The figure shows three views and two pictorial views of one solid part (mm, origin at its lowest corner). Answer the questions. Round coordinates to 2 decimals unless told otherwise and drop trailing zeros. Write each loop counter-clockwise with the first axis right and the second up, starting at its lowest first coordinate (ties: lowest second). Pieces come first, ordered by that corner, then holes. Notation, with made-up numbers: (29, 78) - (60, 78) arc R21 ccw to (60, 94) - close; hole circle Ø5 at (-29, 44.5). An arc over 180 degrees is marked (long way). Answer as CSV lines item,"result". Start each with the question number.
Item 1: A cutting plane is placed at B-B on y = 75. Determine the outline of the cut face in (x, z), and give its area (3 significant figures).
Item 2: A cutting plane is placed at D-D on x = 50. Determine the outline of the cut face in (y, z), and give its area (3 significant figures).
Item 3: Straight lines are drawn through the part: line 1 along X through (y, z) = (75, 1.55); line 2 along Y through (x, z) = (85, 1.3); line 3 along Y through (x, z) = (15, 2.65). For each, find the intervals that lie inside material, in ascending order. Write a range as [from, to].
Item 4: A cutting plane is placed at A-A on z = 4.25. Determine the outline of the cut face in (x, y), and give its area (3 significant figures).
Item 5: Flat-ended cylindrical pins translate along their axes: pin 1 (5.5 mm diameter, centred on x = 15, y = 5, fed in from +Z); pin 2 (3 mm diameter, centred on x = 85, y = 5, fed in from -Z). Find the tip coordinate at first contact, or state that the pin passes through.
Item 6: A cutting plane is placed at C-C on x = 85. Determine the outline of the cut face in (y, z), and give its area (3 significant figures).
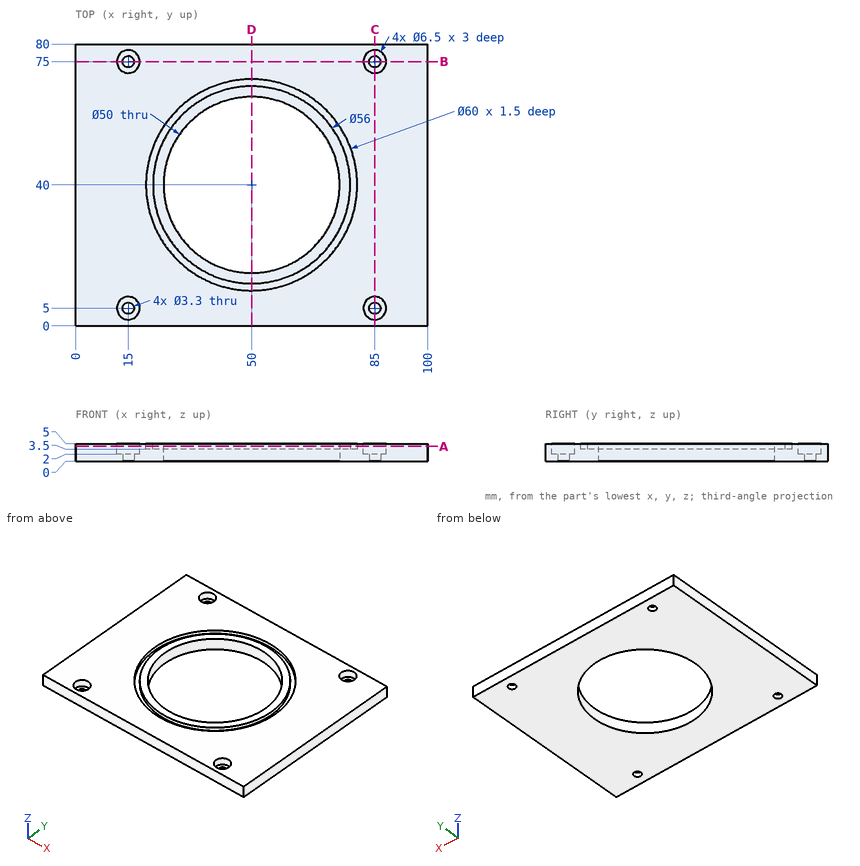
Geometry says:
1,outline,"(0, 0) - (13.35, 0) - (13.35, 2) - (11.75, 2) - (11.75, 5) - (0, 5) - close; (16.65, 0) - (83.35, 0) - (83.35, 2) - (81.75, 2) - (81.75, 5) - (18.25, 5) - (18.25, 2) - (16.65, 2) - close; (86.65, 0) - (100, 0) - (100, 5) - (88.25, 5) - (88.25, 2) - (86.65, 2) - close"
1,area,"448 mm^2"
2,outline,"(0, 0) - (15, 0) - (15, 5) - (12, 5) - (12, 3.5) - (10, 3.5) - (10, 5) - (0, 5) - close; (65, 0) - (80, 0) - (80, 5) - (70, 5) - (70, 3.5) - (68, 3.5) - (68, 5) - (65, 5) - close"
2,area,"144 mm^2"
3,line 1,"x = [0, 13.35], [16.65, 83.35], [86.65, 100]"
3,line 2,"y = [0, 3.35], [6.65, 73.35], [76.65, 80]"
3,line 3,"y = [0, 1.75], [8.25, 71.75], [78.25, 80]"
4,outline,"(0, 0) - (100, 0) - (100, 80) - (0, 80) - close; circle Ø56 at (50, 40); hole circle Ø6.5 at (15, 5); hole circle Ø6.5 at (15, 75); hole circle Ø60 at (50, 40); hole circle Ø50 at (50, 40); hole circle Ø6.5 at (85, 5); hole circle Ø6.5 at (85, 75)"
4,area,"5,540 mm^2"
5,pin 1,"stops at z = 2"
5,pin 2,"passes through"
6,outline,"(0, 0) - (3.35, 0) - (3.35, 2) - (1.75, 2) - (1.75, 5) - (0, 5) - close; (6.65, 0) - (73.35, 0) - (73.35, 2) - (71.75, 2) - (71.75, 5) - (8.25, 5) - (8.25, 2) - (6.65, 2) - close; (76.65, 0) - (80, 0) - (80, 5) - (78.25, 5) - (78.25, 2) - (76.65, 2) - close"
6,area,"348 mm^2"
